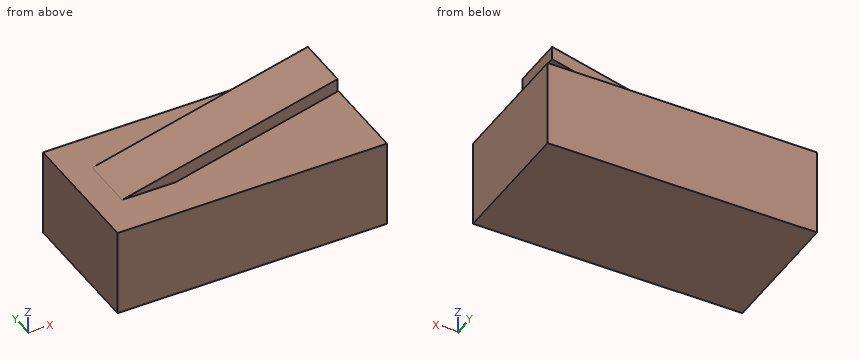
```python
from build123d import *

# Parameters (mm, degrees)
BOITIER_MICROSWITCH_START = -208.5
ESQUISSE1_W               = 20
ESQUISSE1_H               = 10
BOITIER_MICROSWITCH_DEPTH = 6.5
LEVIER_DETECTION_START    = 12
LEVIER_DETECTION_DEPTH    = 4


with BuildPart() as part:
    # Esquisse1 → Boitier_microswitch (new body)
    with BuildSketch(Plane.XY.offset(BOITIER_MICROSWITCH_START)):
        with Locations((0, 14)):
            Rectangle(ESQUISSE1_W, ESQUISSE1_H)
    extrude(amount=-BOITIER_MICROSWITCH_DEPTH)

    # Esquisse2 → Levier_detection (add)
    with BuildSketch(Plane(origin=(0, 0, 0), x_dir=(1, 0, 0), z_dir=(0, 1, 0)).offset(LEVIER_DETECTION_START)):
        Polygon((-8, 208.5), (8, 204.5), (8, 205.5), (-8, 209.5), align=None)
    extrude(amount=LEVIER_DETECTION_DEPTH)


solid = part.part
```
For this review, take the finished solid that the model builds, in its own axes (mm). Give positions to 0.01 mm unless a question says otherwise; leave off trailing zeros. Write each loop counter-clockwise with the first axis right and the second up, starting at its lowest first coordinate (ties: lowest second). Pieces come first, ordered by that corner, then holes. Notation, with made-up numbers: M 31,3 L 49,3 A36 cw 49,38 Z; hole C 13.25,5.5 d7. An arc over 180 degrees is marked long. One line per item, written item: value.
1) Take a section at C-C, the plane z = -208. Write out the cut boundary in (x, y).
Results are:
outline: M -6,12 L -2,12 L -2,16 L -6,16 Z
2) Take a section at D-D, the plane x = 8.75. Write out the cut boundary in (y, z), then the cut area to 3 significant figures.
Results are:
outline: M 9,-215 L 19,-215 L 19,-208.5 L 9,-208.5 Z
area: 65.0 mm²
3) For line 1 (Z direction, x = 3, y = 15.25); line 2 (Z direction, x = 9, y = 10.25); line 3 (Y direction, x = 1.25, z = -207), list the stretches that pass through material, from the lowest coordinate up. Write a range as from..to.
Results are:
line 1: z = -215..-208.5, -206.75..-205.75
line 2: z = -215..-208.5
line 3: y = 12..16
4) Take a section at A-A, the plane x = 3.5. Write out the cut boundary in (y, z) (3 decimals).
Results are:
outline: M 9,-215 L 19,-215 L 19,-208.5 L 9,-208.5 Z; M 12,-206.625 L 16,-206.625 L 16,-205.625 L 12,-205.625 Z
5) For P1, Ø4.5, axis at x = 0.5, z = -205.5, coming from the +Y side; P2, Ø2, axis at x = 2.5, z = -206, coming from the -Y side; P3, Ø3, axis at x = 0.5, y = 13, coming from the +Z side, all flat-tipped, find the tip position at first contact; note any pin that passes through.
Results are:
P1: stops at y = 16
P2: stops at y = 12
P3: stops at z = -206
6) Take a section at B-B, the plane y = 12.75. Write out the cut boundary in (x, z), then the cut area to 3 significant figures.
Results are:
outline: M -10,-215 L 10,-215 L 10,-208.5 L -4,-208.5 L 8,-205.5 L 8,-204.5 L -8,-208.5 L -10,-208.5 Z
area: 144 mm²
